Autodesk Inventor part; units mm, degrees
ref_plane "YZ Plane" through (0, 0, 0) normal (1, 0, 0) x (0, 1, 0)
ref_plane "XZ Plane" through (0, 0, 0) normal (0, 1, 0) x (-1, 0, 0)
ref_plane "XY Plane" through (0, 0, 0) normal (0, 0, 1) x (1, 0, 0)
sketch "草图1" plane through (0, 0, 0) normal (0, 1, 0) x (-1, 0, 0)
  line L0 (8, 25) -> (0, 25)
  line L1 (0, 25) -> (0, 0)
  line L2 (0, 0) -> (8, 0)
  line L3 (8, 0) -> (8, 25)
  circle A0 centre (4, 22.285) radius 1.5
  line L4 (8, 12.5) -> (0, 12.5)
  line L5 (4, 25) -> (4, 0)
  circle A1 centre (4, 2.715) radius 1.5
  dimension "d0" = 25
  dimension "d1" = 8
  dimension "d2" = 3
  dimension "d6" = 19.57
extrude "拉伸1" add sketch "草图1" along normal blind 10 contours L5 A0 | A0 L5 | A1 L5 | L5 A1
extrude "拉伸2" add sketch "草图1" against normal blind 2
properties part number "锁销" material "水"
Geometry: final body of the model. Coordinates: model frame, mm. A direction names the side the tool comes from. Round coordinates to 2 decimals unless told otherwise and drop trailing zeros. Order: outer loops, then holes, each group sorted by start corner. A loop starts at its lowest first (then second) coordinate and runs counter-clockwise, first axis right, second up. Notation, with made-up numbers: (-20, 78.25) -> (23, 78.25) arc R17 ccw to (23, 101.25) -> close; hole circle Ø3 at (77.25, -0.75). An arc over 180 degrees is marked (long way). Use one line per item in the form item = value.
(1) Section A-A on x = -4. Return loops of the section in (y, z) (3 decimals), and give its area (3 significant figures).
Results list:
outline = (-2, 0) -> (0, 0) -> (0, 1.215) -> (10, 1.215) -> (10, 4.215) -> (0, 4.215) -> (0, 20.785) -> (10, 20.785) -> (10, 23.785) -> (0, 23.785) -> (0, 25) -> (-2, 25) -> close
area = 110 mm^2
(2) Access query for faces 5 (the face through (-8, -1, 12)), 6 (the face through (-5.43, 4.93, 2.26)). Directions: +Z, -Z, +X, -X, +Y, -Y. A direction counts if a zero-diameter tool reaches every point of the face in a straight line with its end or side. Return the directions, or none.
Results list:
face_5 = +Z, -Z, -X, +Y, -Y
face_6 = +Y
(3) Section D-D on x = -2.75. Return loops of the section in (y, z).
Results list:
outline = (-2, 0) -> (0, 0) -> (0, 1.89) -> (10, 1.89) -> (10, 3.54) -> (0, 3.54) -> (0, 21.46) -> (10, 21.46) -> (10, 23.11) -> (0, 23.11) -> (0, 25) -> (-2, 25) -> close
(4) First-contact query: pin 1 Ø3 at (x, y) = (-2.5, 3.5) entering from -Z (3 decimals); pin 2 Ø4 at (x, z) = (-6.5, 16) entering from +Y. Flat tips, straight axial feed; report the tip coordinate or a pass-through.
Results list:
pin_1 = 1.215
pin_2 = 0
(5) Ray query, probe 1 along Y at (x, z) = (-0.75, 19); probe 2 along Z at (x, y) = (-3, 7.5); probe 3 along Z at (x, y) = (-4.5, 1.5). Return the intervals inside material, ascending. Write a range as [from, to].
Results list:
probe_1 = [-2, 0]
probe_2 = [1.6, 3.83], [21.17, 23.4]
probe_3 = [1.3, 4.13], [20.87, 23.7]
(6) Draft query along Z for faces 1 (the face through (-4, 10, 22)), 2 (the face through (-4, -1, 0)), 3 (the face through (-4, -1, 25)), 4 (the face through (-4.806, 4.93, 21.02)). Return one class per face: pulls with the +Z half, pulls with the -Z half, needs draft (parallel to the pull), parting line crosses it, or undercut.
Results list:
face_1 = needs draft
face_2 = pulls with the -Z half
face_3 = pulls with the +Z half
face_4 = undercut
(7) Section B-B on z = 15.5. Return loops of the section in (x, y), and give its area (3 significant figures).
Results list:
outline = (-8, -2) -> (0, -2) -> (0, 0) -> (-8, 0) -> close
area = 16.0 mm^2
(8) Section C-C on y = 2.5. Return loops of the section in (x, z) (3 decimals), and give its area (3 significant figures).
Results list:
outline = circle Ø3 at (-4, 2.715); circle Ø3 at (-4, 22.285)
area = 14.1 mm^2
